For this review, take the finished solid that the model builds, in its own axes (mm). A direction names the side the tool comes from. Give positions to 0.01 mm unless a question says otherwise; leave off trailing zeros. Loops run counter-clockwise (first coordinate to the right, second up) from the corner with the lowest first, then second, coordinate; pieces in that order, holes last.
```python
from build123d import *

# Parameters (mm, degrees)
SKETCH1_W                      = 370
SKETCH1_H                      = 114
SKETCH1_R                      = 4
BOSS_EXTRUDE1_DEPTH            = 3
EDGE_FLANGE1_STRIP_W           = 14
EDGE_FLANGE1_STRIP_H           = 3
EDGE_FLANGE1_STRIP_CUT_DEPTH   = 370
EDGE_FLANGE1_STRIP_2_W         = 14
EDGE_FLANGE1_STRIP_2_H         = 3
EDGE_FLANGE1_STRIP_CUT_2_DEPTH = 370
EDGE_FLANGE1_DEPTH             = 370
EDGE_FLANGE1_BEND_DEPTH        = 370
CUT_EXTRUDE2_START             = -185
CUT_EXTRUDE2_DEPTH             = 28
CUT_EXTRUDE2_START_2           = 157
CUT_EXTRUDE2_2_DEPTH           = 28


# Read off the part's stored shape, not the designer's step: Cut-Extrude2
# Sheet-metal steps are written as plain solids
with BuildPart() as part:
    # Sketch1 → Boss-Extrude1 (new body)
    with BuildSketch(Plane(origin=(0, 0, 0), x_dir=(1, 0, 0), z_dir=(0, 1, 0))):
        Rectangle(SKETCH1_W, SKETCH1_H)
        with Locations(Location((-28.284271247, 28.284271247, 0), (0, 0, 270))):
            Circle(SKETCH1_R, mode=Mode.SUBTRACT)
        with Locations(Location((28.284271247, 28.284271247, 0), (0, 0, 270))):
            Circle(SKETCH1_R, mode=Mode.SUBTRACT)
        with Locations(Location((28.284271247, -28.284271247, 0), (0, 0, 270))):
            Circle(SKETCH1_R, mode=Mode.SUBTRACT)
        with Locations(Location((-28.284271247, -28.284271247, 0), (0, 0, 270))):
            Circle(SKETCH1_R, mode=Mode.SUBTRACT)
    extrude(amount=BOSS_EXTRUDE1_DEPTH)

    # Edge-Flange1 strip (across the edge) → Edge-Flange1 strip cut (cut)
    with BuildSketch(Plane(origin=(185, 0, 57), x_dir=(0, 0, -1), z_dir=(-1, 0, 0))):
        with Locations((-6, -1.5)):
            Rectangle(EDGE_FLANGE1_STRIP_W, EDGE_FLANGE1_STRIP_H)
    extrude(amount=EDGE_FLANGE1_STRIP_CUT_DEPTH, mode=Mode.SUBTRACT)

    # Edge-Flange1 strip 2 (across the edge) → Edge-Flange1 strip cut 2 (cut)
    with BuildSketch(Plane(origin=(-185, 0, -57), x_dir=(0, 0, 1), z_dir=(1, 0, 0))):
        with Locations((-6, -1.5)):
            Rectangle(EDGE_FLANGE1_STRIP_2_W, EDGE_FLANGE1_STRIP_2_H)
    extrude(amount=EDGE_FLANGE1_STRIP_CUT_2_DEPTH, mode=Mode.SUBTRACT)

    # Edge-Flange1 section (across the edge) → Edge-Flange1 (add)
    with BuildSketch(Plane(origin=(185, 0, 57), x_dir=(0, 0, -1), z_dir=(-1, 0, 0))):
        with BuildLine():
            Line((-3, 1), (-3, 22))
            Line((-3, 22), (0, 22))
            Line((0, 22), (0, 1))
            ThreePointArc((0, 1), (0.292893219, 0.292893219), (1, 0))
            Line((1, 0), (1, -3))
            ThreePointArc((1, -3), (-1.828427125, -1.828427125), (-3, 1))
        make_face()
    extrude(amount=EDGE_FLANGE1_DEPTH)

    # Edge-Flange1 section 2 (across the edge) → Edge-Flange1 bend (add)
    with BuildSketch(Plane(origin=(-185, 0, -57), x_dir=(0, 0, 1), z_dir=(1, 0, 0))):
        with BuildLine():
            Line((-3, 1), (-3, 22))
            Line((-3, 22), (0, 22))
            Line((0, 22), (0, 1))
            ThreePointArc((0, 1), (0.292893219, 0.292893219), (1, 0))
            Line((1, 0), (1, -3))
            ThreePointArc((1, -3), (-1.828427125, -1.828427125), (-3, 1))
        make_face()
    extrude(amount=EDGE_FLANGE1_BEND_DEPTH)

    # Cut-Extrude2 outline → Cut-Extrude2 (cut)
    with BuildSketch(Plane.YZ.offset(CUT_EXTRUDE2_START)):
        with BuildLine():
            ThreePointArc((-1, -60), (1.828427125, -58.828427125), (3, -56))
            Line((3, -56), (0, -56))
            ThreePointArc((0, -56), (-0.292893219, -56.707106781), (-1, -57))
            Line((-1, -57), (-22, -57))
            Line((-22, -57), (-22, -60))
            Line((-22, -60), (-1, -60))
        make_face()
        with BuildLine():
            ThreePointArc((-1, 57), (-0.292893219, 56.707106781), (0, 56))
            Line((0, 56), (3, 56))
            ThreePointArc((3, 56), (1.828427125, 58.828427125), (-1, 60))
            Line((-1, 60), (-22, 60))
            Line((-22, 60), (-22, 57))
            Line((-22, 57), (-1, 57))
        make_face()
    extrude(amount=CUT_EXTRUDE2_DEPTH, mode=Mode.SUBTRACT)

    # Cut-Extrude2 2 outline → Cut-Extrude2 2 (cut)
    with BuildSketch(Plane.YZ.offset(CUT_EXTRUDE2_START_2)):
        with BuildLine():
            ThreePointArc((-1, -60), (1.828427125, -58.828427125), (3, -56))
            Line((3, -56), (0, -56))
            ThreePointArc((0, -56), (-0.292893219, -56.707106781), (-1, -57))
            Line((-1, -57), (-22, -57))
            Line((-22, -57), (-22, -60))
            Line((-22, -60), (-1, -60))
        make_face()
        with BuildLine():
            ThreePointArc((-1, 57), (-0.292893219, 56.707106781), (0, 56))
            Line((0, 56), (3, 56))
            ThreePointArc((3, 56), (1.828427125, 58.828427125), (-1, 60))
            Line((-1, 60), (-22, 60))
            Line((-22, 60), (-22, 57))
            Line((-22, 57), (-1, 57))
        make_face()
    extrude(amount=CUT_EXTRUDE2_2_DEPTH, mode=Mode.SUBTRACT)


solid = part.part
```
Item 1: Take a section at A-A on y = -4.25. Give the boundary of the cut face in (x, z), and give its area (3 significant figures).
Answer:
outline: (-157, -60) - (157, -60) - (157, -57) - (-157, -57) - close; (-157, 57) - (157, 57) - (157, 60) - (-157, 60) - close
area: 1,880 mm2
Item 2: Take a section at C-C on z = 37.5. Give the boundary of the cut face in (x, y).
Answer:
outline: (-185, 0) - (185, 0) - (185, 3) - (-185, 3) - close
Item 3: Take a section at B-B on x = 115.5. Give the boundary of the cut face in (y, z).
Answer:
outline: (-22, -60) - (-1, -60) arc R4 ccw to (3, -56) - (3, 56) arc R4 ccw to (-1, 60) - (-22, 60) - (-22, 57) - (-1, 57) arc R1 cw to (0, 56) - (0, -56) arc R1 cw to (-1, -57) - (-22, -57) - close
Item 4: Tool access review of faces 1 (the flat face through (-3, 0, -1)), 2 (the cylindrical face through (-29.816, 1.479, 31.979)): name each direction out of +Z, -Z, +X, -X, +Y, -Y from which nothing blocks a thin tool from reaching the whole face with its end or side.
Answer:
face 1: +X, -X, -Y
face 2: +Y, -Y
Item 5: The part is to be moulded in two halves that separate along Z. For faces 3 (the cylindrical face through (-28.11, 1.48, -32.28)), 4 (the flat face through (2, -11, 60)), 5 (the flat face through (-3, 3, -1)), say which applies: released by +Z, released by -Z, zero draft, split by the parting line, or undercut.
Answer:
face 3: undercut
face 4: released by +Z
face 5: zero draft
Item 6: For L1, parallel to Z at x = 66.5, y = -3.25; L2, parallel to Y at x = -70.5, z = -5; L3, parallel to Z at x = 72.5, y = 1, list the stretches that pass through material, from the lowest coordinate up.
Answer:
L1: z = -60 to -57, 57 to 60
L2: y = 0 to 3
L3: z = -59.46 to 59.46
Item 7: Clearance check with flat-ended pins moving along their axes: pin 1 Ø3.5 at (x, y) = (-164, 2) entering from +Z; pin 2 Ø2 at (y, z) = (-13.5, -58) entering from -X; pin 3 Ø3 at (x, y) = (12.5, -0.5) entering from +Z; pin 4 Ø3.5 at (x, y) = (170.5, 2) entering from -Z. State where each tip first meets the part, or that it passes through.
Answer:
pin 1: stops at z = 56
pin 2: stops at x = -157
pin 3: stops at z = 60
pin 4: stops at z = -56
